For this review, take the finished solid that the model builds, in its own axes (mm). Face numbers are marked on the shaded views. A direction names the side the tool comes from. Coordinates: 2 decimals unless noted, no trailing zeros. Write each loop counter-clockwise with the first axis right and the second up, starting at its lowest first coordinate (ties: lowest second). Pieces come first, ordered by that corner, then holes. Notation, with made-up numbers: (77.25, 53.25) - (114.25, 53.25) arc R16 ccw to (114.25, 79.25) - close; hole circle Ø7 at (50, -8.75). An arc over 180 degrees is marked (long way). Write each question's results on one line, items separated by ' | '.
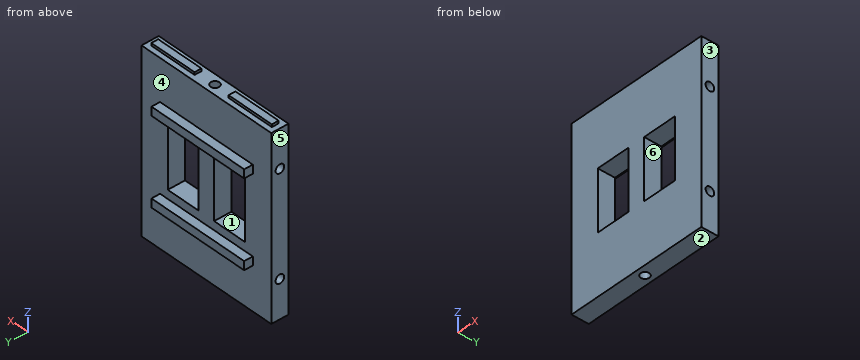
Autodesk Fusion 360 part; units mm, degrees
sketch "Sketch1" plane through (0, 0, 0) normal (0, 1, 0) x (1, 0, 0)
  line L0 (0, 0) -> (42, 0)
  line L1 (0, 0) -> (-42, 0)
  line L2 (-42, 0) -> (-42, -104)
  line L3 (42, 0) -> (42, -104)
  line L4 (-42, -104) -> (42, -104)
  dimension "d1" = 42
  dimension "d2" = 42
  dimension "d3" = 104
  dimension "d4" = 104
extrude "Extrude1" add sketch "Sketch1" along normal blind 10
sketch "Sketch2" plane through (-42, 0, 0) normal (-1, 0, 0) x (0, 0, 1)
  line L0 (0, 0) -> (104, 0)
  line L1 (104, 0) -> (104, 10)
  line L2 (104, 10) -> (0, 10)
  line L3 (0, 10) -> (0, 0)
sketch "Sketch3" plane through (0, 0, 104) normal (0, 0, 1) x (1, 0, 0)
  line L0 (-42, 0) -> (42, 0)
  line L1 (42, 0) -> (42, 10)
  line L2 (42, 10) -> (-42, 10)
  line L3 (-42, 10) -> (-42, 0)
sketch "Sketch4" plane through (0, 0, 104) normal (0, 0, 1) x (1, 0, 0)
sketch "Sketch5" plane through (0, 0, 104) normal (0, 0, 1) x (1, 0, 0)
sketch "Sketch6" plane through (0, 0, 104) normal (0, 0, 1) x (1, 0, 0)
  line L0 (-39, 7) -> (-39, 3)
  line L1 (-39, 3) -> (-11, 3)
  line L2 (-11, 3) -> (-11, 7)
  line L3 (-11, 7) -> (-39, 7)
  dimension "d21" = 28
sketch "Sketch7" plane through (0, 0, 104) normal (0, 0, 1) x (1, 0, 0)
  line L0 (39, 5) -> (39, 3)
  line L1 (39, 3) -> (11, 3)
  line L2 (11, 3) -> (11, 7)
  line L3 (11, 7) -> (39, 7)
  line L4 (39, 7) -> (39, 5)
  circle A0 centre (0, 5) radius 2.5
  dimension "d22" = 28
  dimension "d23" = 5
extrude "Extrude2" add sketch "Sketch6" sketch "Sketch7" along normal blind 1.5 of sketch 2 contours L0 L1 L2 L3 L4
sketch "Sketch8" plane through (0, 0, 104) normal (0, 0, 1) x (1, 0, 0)
  circle A0 centre (0, 5) radius 2.5
  dimension "d26" = 5
extrude "Extrude3" cut sketch "Sketch8" against normal blind 25
sketch "Sketch9" plane through (0, 0, 0) normal (0, 0, -1) x (-1, 0, 0)
  line L0 (-42, 0) -> (42, 0)
  line L1 (42, 0) -> (42, 10)
  line L2 (42, 10) -> (-42, 10)
  line L3 (-42, 10) -> (-42, 0)
  circle A0 centre (0, 5) radius 2.5
  dimension "d29" = 5
extrude "Extrude4" cut sketch "Sketch9" against normal blind 25 contours A0
sketch "Sketch10" plane through (42, 0, 0) normal (1, 0, 0) x (0, 0, -1)
  line L0 (-104, 0) -> (0, 0)
  line L1 (0, 0) -> (0, 10)
  line L2 (0, 10) -> (-104, 10)
  line L3 (-104, 10) -> (-104, 0)
  circle A0 centre (-79, 5) radius 2.5
  circle A1 centre (-22, 5) radius 2.5
  dimension "d33" = 5
  dimension "d35" = 5
extrude "Extrude5" cut sketch "Sketch10" against normal blind 25 contours A0 | A1
sketch "Sketch11" plane through (-42, 0, 0) normal (-1, 0, 0) x (0, 0, 1)
  circle A0 centre (22, 5) radius 2.5
  circle A1 centre (82, 5) radius 2.5
  dimension "d39" = 5
  dimension "d41" = 5
extrude "Extrude6" cut sketch "Sketch11" against normal blind 25
sketch "Sketch12" plane through (0, 10, 0) normal (0, 1, 0) x (-1, 0, 0)
  line L0 (-42, 0) -> (42, 0)
  line L1 (42, 0) -> (42, 104)
  line L2 (42, 104) -> (-42, 104)
  line L3 (-42, 104) -> (-42, 0)
sketch "Sketch13" plane through (0, 10, 0) normal (0, 1, 0) x (-1, 0, 0)
  line L0 (-30, 80) -> (-30, 75)
  line L1 (-30, 75) -> (30, 75)
  line L2 (30, 75) -> (30, 80)
  line L3 (30, 80) -> (-30, 80)
  line L4 (-30, 30) -> (30, 30)
  line L5 (30, 30) -> (30, 25)
  line L6 (30, 25) -> (-30, 25)
  line L7 (-30, 25) -> (-30, 30)
  dimension "d44" = 5
  dimension "d45" = 5
extrude "Extrude7" add sketch "Sketch13" along normal blind 5
sketch "Sketch14" plane through (0, 10, 0) normal (0, 1, 0) x (-1, 0, 0)
  line L0 (25, 35) -> (5, 35)
  line L1 (5, 35) -> (5, 70)
  line L2 (5, 70) -> (25, 70)
  line L3 (25, 70) -> (25, 35)
  line L4 (-5, 35) -> (-25, 35)
  line L5 (-25, 35) -> (-25, 70)
  line L6 (-25, 70) -> (-5, 70)
  line L7 (-5, 70) -> (-5, 35)
extrude "Extrude8" cut sketch "Sketch14" against normal blind 20
Q1. For pin 1 (1.2 mm diameter, centred on x = 22, z = 105, fed in from +Y); pin 2 (1.5 mm diameter, centred on y = 6, z = 21, fed in from +X); pin 3 (1.5 mm diameter, centred on y = 12.5, z = 78.5, fed in from -X), all flat-tipped, find the tip position at first contact; note any pin that passes through.
Results found:
pin 1: y = 7 | pin 2: x = 17 | pin 3: x = -30
Q2. Take a section at B-B on x = 8. State the section outline as (y, z) points, plus the area to 3 significant figures.
Results found:
outline: (0, 0) - (10, 0) - (10, 25) - (15, 25) - (15, 30) - (10, 30) - (10, 35) - (0, 35) - close; (0, 70) - (10, 70) - (10, 75) - (15, 75) - (15, 80) - (10, 80) - (10, 104) - (0, 104) - close | area: 740 mm2
Q3. For the marked faces 1 and 2, list the 3-axis set-ups (+Z, -Z, +X, -X, +Y, -Y) from which the entire face can be reached by the end or side of a thin tool; tool diameter is ignored.
Results found:
face 1: +Y, -Y | face 2: -Z, +X, -X, +Y, -Y
Q4. Mouldability with a two-part tool opening along X and no side actions: class the marked faces 3, 4, 5 and 6 as pulls with the +X half, pulls with the -X half, needs draft (parallel to the pull), parting line crosses it, or undercut.
Results found:
face 3: pulls with the +X half | face 4: needs draft | face 5: pulls with the -X half | face 6: undercut
Q5. Take a section at C-C on y = 13.25. State the section outline as (x, z) points, plus the area to 3 significant figures.
Results found:
outline: (-30, 25) - (30, 25) - (30, 30) - (-30, 30) - close; (-30, 75) - (30, 75) - (30, 80) - (-30, 80) - close | area: 600 mm2
Q6. Take a section at A-A on z = 66. State the section outline as (x, y) points, plus the area to 3 significant figures.
Results found:
outline: (-42, 0) - (-25, 0) - (-25, 10) - (-42, 10) - close; (-5, 0) - (5, 0) - (5, 10) - (-5, 10) - close; (25, 0) - (42, 0) - (42, 10) - (25, 10) - close | area: 440 mm2
Q7. Wall thickness on line 1 along X through (y, z) = (7.5, 41); line 2 along X through (y, z) = (5.25, 97.5); line 3 along Z through (x, y) = (-6, 9): over which ranges is each line inside the solid? List them lowest first. Write a range as from..to.
Results found:
line 1: -42..-25, -5..5, 25..42 | line 2: -42..-2.49, 2.49..42 | line 3: 0..35, 70..104
Q8. Take a section at D-D on z = 22. State the section outline as (x, y) points.
Results found:
outline: (-42, 0) - (42, 0) - (42, 2.5) - (17, 2.5) - (17, 7.5) - (42, 7.5) - (42, 10) - (-42, 10) - (-42, 7.5) - (-17, 7.5) - (-17, 2.5) - (-42, 2.5) - close; hole circle Ø5 at (0, 5)
